```python
from build123d import *

# Parameters (mm, degrees)
SKETCH_2_W          = 40
SKETCH_2_H          = 40
SKETCH_2_R          = 2
EXTRUDE_1_DEPTH     = 1.2
SKETCH_3_W          = 40
SKETCH_3_H          = 47
EXTRUDE_2_DEPTH     = 1.2
FILLET_1_R          = 1
FILLET_2_R          = 20
FILLET_3_R          = 2
CUT_EXTRUDE_1_DEPTH = 75.20539064
SKETCH_7_R          = 2
CUT_EXTRUDE_3_DEPTH = 75.20539064
FILLET_4_R          = 0.2


with BuildPart() as part:
    # 草图2 → 凸台-拉伸1 (new body)
    with BuildSketch(Plane.XY):
        with Locations((20, 20)):
            Rectangle(SKETCH_2_W, SKETCH_2_H)
        with Locations((5, 32)):
            Circle(SKETCH_2_R, mode=Mode.SUBTRACT)
        with Locations((35, 8)):
            Circle(SKETCH_2_R, mode=Mode.SUBTRACT)
        with Locations((5, 8)):
            Circle(SKETCH_2_R, mode=Mode.SUBTRACT)
        with Locations((35, 32)):
            Circle(SKETCH_2_R, mode=Mode.SUBTRACT)
    extrude(amount=EXTRUDE_1_DEPTH)

    # 草图3 → 凸台-拉伸2 (add)
    with BuildSketch(Plane(origin=(0, 40, 0), x_dir=(1, 0, 0), z_dir=(0, 1, 0))):
        with Locations((20, -23.5)):
            Rectangle(SKETCH_3_W, SKETCH_3_H)
    extrude(amount=EXTRUDE_2_DEPTH)

    # 圆角1
    fillet_1_edges = [part.edges().sort_by_distance(p)[0] for p in [
        (20, 40, 1.2),
        (20, 41.2, 0),
    ]]
    fillet(fillet_1_edges, radius=FILLET_1_R)

    # 圆角2
    fillet_2_edges = [part.edges().sort_by_distance(p)[0] for p in [
        (0, 40.6, 47),
        (40, 40.6, 47),
    ]]
    fillet(fillet_2_edges, radius=FILLET_2_R - 0.0001)  # a hair under: the kernel refuses the full size

    # 圆角3
    fillet_3_edges = [part.edges().sort_by_distance(p)[0] for p in [
        (40, 0, 0.6),
        (0, 0, 0.6),
    ]]
    fillet(fillet_3_edges, radius=FILLET_3_R)

    # 草图5 → 切除-拉伸1 (cut, through all)
    with BuildSketch(Plane(origin=(0, 41.2, 0), x_dir=(1, 0, 0), z_dir=(0, 1, 0))):
        with BuildLine():
            Line((26.5, -19.75), (26.5, -34.25))
            ThreePointArc((26.5, -34.25), (20, -40.75), (13.5, -34.25))
            Line((13.5, -34.25), (13.5, -19.75))
            ThreePointArc((13.5, -19.75), (20, -13.25), (26.5, -19.75))
        make_face()
    extrude(amount=-CUT_EXTRUDE_1_DEPTH, mode=Mode.SUBTRACT)

    # 草图7 → 切除-拉伸3 (cut, through all)
    with BuildSketch(Plane(origin=(0, 41.2, 0), x_dir=(1, 0, 0), z_dir=(0, 1, 0))):
        with Locations(Location((36, -27, 0), (0, 0, 270))):
            Circle(SKETCH_7_R)
        with Locations(Location((4, -27, 0), (0, 0, 270))):
            Circle(SKETCH_7_R)
        with Locations(Location((28, -40.856406461, 0), (0, 0, 270))):
            Circle(SKETCH_7_R)
        with Locations(Location((12, -40.856406461, 0), (0, 0, 270))):
            Circle(SKETCH_7_R)
        with Locations(Location((28, -13.143593539, 0), (0, 0, 270))):
            Circle(SKETCH_7_R)
        with Locations(Location((12, -13.143593539, 0), (0, 0, 270))):
            Circle(SKETCH_7_R)
    extrude(amount=-CUT_EXTRUDE_3_DEPTH, mode=Mode.SUBTRACT)

    # 圆角4
    fillet_4_edges = [part.edges().sort_by_distance(p)[0] for p in [
        (20, 40, 13.25),
        (26.5, 40, 27),
        (20, 40, 40.75),
        (13.5, 40, 27),
        (20, 41.2, 13.25),
        (13.5, 41.2, 27),
        (20, 41.2, 40.75),
        (26.5, 41.2, 27),
    ]]
    fillet(fillet_4_edges, radius=FILLET_4_R)


solid = part.part
```
Part model, mm, in its own coordinate system. A direction names the side the tool comes from. Round coordinates to 2 decimals unless told otherwise and drop trailing zeros. Write each loop counter-clockwise with the first axis right and the second up, starting at its lowest first coordinate (ties: lowest second). Pieces come first, ordered by that corner, then holes. Notation, with made-up numbers: (4.25, 64) -> (52.25, 64) arc R25 ccw to (52.25, 89) -> close; hole circle Ø11 at (51.5, 23). An arc over 180 degrees is marked (long way). Return JSON: item names as keys, results as strings. Group by question number.
Q1. Pin check, flat tips, straight feed: pin 1 (2 mm diameter, centred on x = 15, y = 30, fed in from +Z); pin 2 (20 mm diameter, centred on x = 26, z = 24, fed in from -Y). Stop position of each tip, or through.
Q2. Saw through at C-C on x = 28. Write the cut outline in (y, z), plus the area to 3 significant figures.
Q3. Probe L1, parallel to X at y = 40.9, z = 27; L2, parallel to Y at x = 5, z = 0.35; L3, parallel to Y at x = 6, z = 10. List the from-to ranges inside material, lowest first. Write a range as [from, to].
Q4. Saw through at B-B on x = 35. Write the cut outline in (y, z).
Q5. Saw through at D-D on y = 15. Write the cut outline in (x, z).
Q6. Mould opens along X. For faces 1 (the flat face through (15, 40, 14)), 2 (the cylindrical face through (26.226, 40.608, 41.779)), 3 (the cylindrical face through (0.57, 0.6, 0.61)) say: pulls with the +X half, pulls with the -X half, needs draft (parallel to the pull), parting line crosses it, or undercut.
Q7. Which spindle directions (+Z, -Z, +X, -X, +Y, -Y) get a long thin tool onto all of the face, cutting with end or side? Do faces 4 (the flat face through (20, 20, 1.2)), 5 (the cylindrical face through (5.703, 40.608, 40.986)), 6 (the cylindrical face through (19.86, 40.61, 13.25)). Say none if no direction does.
Q8. Saw through at A-A on y = 8. Write the cut outline in (x, z).
Answer:
{
 "1": {"pin 1": "z = 1.2", "pin 2": "y = 40"},
 "2": {"outline": "(0, 0) -> (40.2, 0) arc R1 ccw to (41.2, 1) -> (41.2, 11.14) -> (40, 11.14) -> (40, 2.2) arc R1 cw to (39, 1.2) -> (0, 1.2) -> close; (40, 15.14) -> (41.2, 15.14) -> (41.2, 38.86) -> (40, 38.86) -> close; (40, 42.86) -> (41.2, 42.86) -> (41.2, 45.33) -> (40, 45.33) -> close", "area": "92.8 mm2"},
 "3": {"L1": "[0, 2], [6, 13.5], [26.5, 34], [38, 40]", "L2": "[0, 6], [10, 30], [34, 40.96]", "L3": "[40, 41.2]"},
 "4": {"outline": "(0, 0) -> (6, 0) -> (6, 1.2) -> (0, 1.2) -> close; (10, 0) -> (30, 0) -> (30, 1.2) -> (10, 1.2) -> close; (34, 0) -> (40.2, 0) arc R1 ccw to (41.2, 1) -> (41.2, 25.27) -> (40, 25.27) -> (40, 2.2) arc R1 cw to (39, 1.2) -> (34, 1.2) -> close; (40, 28.73) -> (41.2, 28.73) -> (41.2, 40.23) -> (40, 40.23) -> close"},
 "5": {"outline": "(0, 0) -> (40, 0) -> (40, 1.2) -> (0, 1.2) -> close"},
 "6": {"face 1": "needs draft", "face 2": "undercut", "face 3": "pulls with the -X half"},
 "7": {"face 4": "+Z, +X, -X, -Y", "face 5": "+Z, -X, +Y, -Y", "face 6": "+Y, -Y"},
 "8": {"outline": "(0, 0) -> (3, 0) -> (3, 1.2) -> (0, 1.2) -> close; (7, 0) -> (33, 0) -> (33, 1.2) -> (7, 1.2) -> close; (37, 0) -> (40, 0) -> (40, 1.2) -> (37, 1.2) -> close"}
}
